from build123d import *

# Parameters (mm, degrees)
EXTRUDE_1_DEPTH = 40
FILLET_1_R      = 1
FILLET_2_R      = 10
FILLET_3_R      = 10
SHELL_START     = 1
SHELL_1_DEPTH   = 38


# Read off the part's stored shape, not the designer's step: 抽壳1
with BuildPart() as part:
    # 草图1 → 凸台-拉伸1 (new body)
    with BuildSketch(Plane.XY):
        with BuildLine():
            Line((-40, -106.75), (40, -106.75))
            Line((40, -106.75), (40, -96.75))
            Line((40, -96.75), (20.152543264, -96.75))
            Line((20.152543264, -96.75), (20.152543264, -20.152543264))
            ThreePointArc((20.152543264, -20.152543264), (0, -28.5), (-20.152543264, -20.152543264))
            Line((-20.152543264, -20.152543264), (-20.152543264, -96.75))
            Line((-20.152543264, -96.75), (-40, -96.75))
            Line((-40, -96.75), (-40, -106.75))
        make_face()
    extrude(amount=EXTRUDE_1_DEPTH)

    # 圆角1
    fillet_1_edges = [part.edges().sort_by_distance(p)[0] for p in [
        (-20.152543264, -20.152543264, 20),
        (20.152543264, -20.152543264, 20),
    ]]
    fillet(fillet_1_edges, radius=FILLET_1_R)

    # 圆角2
    fillet_2_edges = [part.edges().sort_by_distance(p)[0] for p in [
        (40, -96.75, 20),
        (-40, -96.75, 20),
    ]]
    fillet(fillet_2_edges, radius=FILLET_2_R - 0.0001)  # a hair under: the kernel refuses the full size

    # 圆角3
    fillet_3_edges = [part.edges().sort_by_distance(p)[0] for p in [
        (20.152543264, -96.75, 20),
        (-20.152543264, -96.75, 20),
    ]]
    fillet(fillet_3_edges, radius=FILLET_3_R)

    # 抽壳1 outline → 抽壳1 (cut)
    with BuildSketch(Plane.XY.offset(SHELL_START)):
        with BuildLine():
            Line((19.152543264, -86.750581745), (19.152543264, -22.437247749))
            ThreePointArc((19.152543264, -22.437247749), (0, -29.5), (-19.152543264, -22.437247749))
            Line((-19.152543264, -22.437247749), (-19.152543264, -86.750581745))
            ThreePointArc((-19.152543264, -86.750581745), (-22.344762313, -94.499036857), (-30.068644469, -97.750261785))
            ThreePointArc((-30.068644469, -97.750261785), (-36.388184414, -100.410354908), (-39, -106.75))
            Line((-39, -106.75), (39, -106.75))
            ThreePointArc((39, -106.75), (36.388184414, -100.410354908), (30.068644469, -97.750261785))
            ThreePointArc((30.068644469, -97.750261785), (22.344762313, -94.499036857), (19.152543264, -86.750581745))
        make_face()
    extrude(amount=SHELL_1_DEPTH, mode=Mode.SUBTRACT)


solid = part.part
Design review of the part built by this model. Coordinates are the model's own, in mm. A direction names the side the tool comes from. Coordinates: 2 decimals unless noted, no trailing zeros. Order: outer loops, then holes, each group sorted by start corner. A loop starts at its lowest first (then second) coordinate and runs counter-clockwise, first axis right, second up.
Item 1: Take a section at B-B, the plane x = -7.5. Write out the cut boundary in (y, z), then the cut area to 3 significant figures.
Item 2: The part is to be moulded in two halves that separate along X. For faces 1 (the flat face through (-20.153, -54, 20)), 2 (the flat face through (-0.2, -106.75, 0.6)), 3 (the cylindrical face through (22.43, -94.584, 19.734)), say which applies: pulls with the +X half, pulls with the -X half, needs draft (parallel to the pull), parting line crosses it, or undercut.
Item 3: For line 1 (Z direction, x = 2, y = -31); line 2 (X direction, y = -63.5, z = 22.5); line 3 (X direction, y = -25, z = 27), list the stretches that pass through material, from the lowest coordinate up.
Item 4: Take a section at C-C, the plane x = 5. Write out the cut boundary in (y, z), then the cut area to 3 significant figures.
Item 5: For pin 1 Ø1 at (y, z) = (-74.5, 12) entering from -X; pin 2 Ø6 at (x, z) = (-11.5, 7.5) entering from -Y; pin 3 Ø2 at (y, z) = (-82.5, 34.5) entering from +X, all flat-tipped, find the tip position at first contact; note any pin that passes through.
Item 6: For faces 4 (the flat face through (-19.153, -54, 20)), 5 (the cylindrical face through (0.3, -28.5, 19.7)), 6 (the flat face through (20.153, -55, 20)), list the 3-axis set-ups (+Z, -Z, +X, -X, +Y, -Y) from which the entire face can be reached by the end or side of a thin tool; tool diameter is ignored.
Item 7: Take a section at A-A, the plane y = -54. Write out the cut boundary in (x, z).
The answers:
1. outline: (-106.75, 0) - (-27.5, 0) - (-27.5, 40) - (-106.75, 40) - (-106.75, 39) - (-28.53, 39) - (-28.53, 1) - (-106.75, 1) - close
1. area: 198 mm2
2. face 1: pulls with the -X half
2. face 2: needs draft
2. face 3: undercut
3. line 1: z = 0 to 1, 39 to 40
3. line 2: x = -20.15 to -19.15, 19.15 to 20.15
3. line 3: x = -20.15 to -19.15, -15.66 to -13.68, 13.68 to 15.66, 19.15 to 20.15
4. outline: (-106.75, 0) - (-28.06, 0) - (-28.06, 40) - (-106.75, 40) - (-106.75, 39) - (-29.07, 39) - (-29.07, 1) - (-106.75, 1) - close
4. area: 196 mm2
5. pin 1: stops at x = -20.15
5. pin 2: stops at y = -28.25
5. pin 3: stops at x = 20.15
6. face 4: -Y
6. face 5: +Z, -Z, +Y
6. face 6: +Z, -Z, +X, +Y
7. outline: (-20.15, 0) - (20.15, 0) - (20.15, 40) - (-20.15, 40) - close; hole (-19.15, 1) - (19.15, 1) - (19.15, 39) - (-19.15, 39) - close
